Here's how the part is built. I have some questions about the finished solid (model axes, mm). A direction names the side the tool comes from. Round coordinates to 2 decimals unless told otherwise and drop trailing zeros. Order: outer loops, then holes, each group sorted by start corner. A loop starts at its lowest first (then second) coordinate and runs counter-clockwise, first axis right, second up.
```python
from build123d import *

# Parameters (mm, degrees)
F0_W     = 180
F0_H     = 50
F1_DEPTH = 50
F2_T     = -2.5
F0_W_2   = 190
F0_H_2   = 60
F3_DEPTH = 8
F5_DEPTH = 1.75


with BuildPart() as f1:
    # F0 (on Top) → F1 (new body)
    with BuildSketch(Plane.XY):
        with Locations((42.104505, 8.436477)):
            Rectangle(F0_W, F0_H)
    extrude(amount=F1_DEPTH)

    # F2
    f2_openings = [f1.faces().sort_by_distance(p)[0] for p in [
        (42.104505, 8.436477, 50),
    ]]
    offset(amount=F2_T, openings=f2_openings)

    # F0 (on Top) → F3 (join)
    with BuildSketch(Plane.XY):
        with Locations((42.104505, 8.436477)):
            Rectangle(F0_W_2, F0_H_2)
        with Locations((42.104505, 8.436477)):
            Rectangle(F0_W, F0_H, mode=Mode.SUBTRACT)
    extrude(amount=F3_DEPTH)

    # F4 (on face) → F5 (cut)
    with BuildSketch(Plane.XZ.offset(16.563523)):
        with BuildLine():
            Line((18.778705, 27.266525), (18.778705, 39.354309))
            Line((18.778705, 39.354309), (14.466432, 39.354309))
            Line((14.466432, 39.354309), (14.466432, 27.266525))
            ThreePointArc((14.466432, 27.266525), (23.398135, 18.334822), (32.329838, 27.266525))
            Line((32.329838, 27.266525), (32.329838, 39.507348))
            Line((32.329838, 39.507348), (27.672919, 39.507348))
            Line((27.672919, 39.507348), (27.672919, 27.266525))
            ThreePointArc((27.672919, 27.266525), (23.225812, 22.819418), (18.778705, 27.266525))
        make_face()
        Polygon((-1.653947, 40.034065), (-6.702017, 40.034065), (-6.702017, 19.841794), (7.721034, 19.841794), (7.721034, 24.168709), (-1.653947, 24.168709), align=None)
        Polygon((48.105575, 40.034065), (41.615201, 40.034065), (41.615201, 19.841794), (48.105575, 19.841794), (48.105575, 26.812933), (55.495456, 19.841794), (63.49016, 19.841794), (53.456086, 28.907086), (63.49016, 40.013472), (55.495456, 40.013472), (48.105575, 32.753399), align=None)
        Polygon((87.829128, 40.034065), (73.290575, 40.034065), (73.290575, 19.841794), (87.829128, 19.841794), (87.829128, 24.375837), (78.053206, 24.375837), (78.053206, 28.907086), (87.829128, 28.907086), (87.829128, 32.753399), (78.053206, 32.753399), (78.053206, 36.157073), (87.829128, 36.157073), align=None)
    extrude(amount=-F5_DEPTH, mode=Mode.SUBTRACT)


solid = f1.part
```
1) If we section it at B-B (y = 1): Write out the boundary of the cut face in (x, z), plus the area to 4 significant figures.
2) If we section it at C-C (x = -41): Write out the boundary of the cut face in (y, z), plus the area to 4 significant figures.
3) I'm going to push flat-ended pins straight in: pin 1 (22.5 mm diameter, centred on y = 16, z = 25.5, fed in from +X); pin 2 (14 mm diameter, centred on x = 3.5, z = 27, fed in from -Y); pin 3 (1 mm diameter, centred on x = 26.5, y = 10, fed in from +Z). Where does each tip first touch, or does it pass through?
4) If we section it at D-D (x = 85.5): Write out the boundary of the cut face in (y, z), plus the area to 3 significant figures.
5) We'd pull the mould along Y, two halves only. Please class faces 5 (the flat face through (129.605, 8, 26)), 6 (the flat face through (41, 38.436, 4)), 7 (the flat face through (41, -14.064, 26)), 8 (the flat face through (-47.895, 8, 29)): +Y half, -Y half, draft (parallel to the pull), parting line (faces both ways), or undercut.
6) For faces 1 (the flat face through (41, 33.436, 29)), 2 (the flat face through (137.105, 8, 4)), 3 (the cylindrical face through (23.202, -15.701, 18.337)), 4 (the flat face through (-45.395, 8, 26)), which set-ups out of +Z, -Z, +X, -X, +Y, -Y let a thin tool reach every point of the face, with its end or its side?
7) I need wall thicknesses on line 1 (Y direction, x = 123, z = 19); line 2 (Y direction, x = -26.5, z = 4); line 3 (X direction, y = -1.5, z = 22). Which ranges of each line are inside material? Lowest first, please.
8) If we section it at A-A (x = 3): Write out the boundary of the cut face in (y, z), plus the area to 3 significant figures.
Solutions:
1. outline: (-52.9, 0) - (137.1, 0) - (137.1, 8) - (132.1, 8) - (132.1, 50) - (129.6, 50) - (129.6, 2.5) - (-45.4, 2.5) - (-45.4, 50) - (-47.9, 50) - (-47.9, 8) - (-52.9, 8) - close
1. area: 767.5 mm2
2. outline: (-21.56, 0) - (38.44, 0) - (38.44, 8) - (33.44, 8) - (33.44, 50) - (30.94, 50) - (30.94, 2.5) - (-14.06, 2.5) - (-14.06, 50) - (-16.56, 50) - (-16.56, 8) - (-21.56, 8) - close
2. area: 442.5 mm2
3. pin 1: stops at x = 132.1
3. pin 2: stops at y = -16.56
3. pin 3: stops at z = 2.5
4. outline: (-21.56, 0) - (38.44, 0) - (38.44, 8) - (33.44, 8) - (33.44, 50) - (30.94, 50) - (30.94, 2.5) - (-14.06, 2.5) - (-14.06, 50) - (-16.56, 50) - (-16.56, 40.03) - (-14.81, 40.03) - (-14.81, 36.16) - (-16.56, 36.16) - (-16.56, 32.75) - (-14.81, 32.75) - (-14.81, 28.91) - (-16.56, 28.91) - (-16.56, 24.38) - (-14.81, 24.38) - (-14.81, 19.84) - (-16.56, 19.84) - (-16.56, 8) - (-21.56, 8) - close
4. area: 421 mm2
5. face 5: undercut
5. face 6: +Y half
5. face 7: undercut
5. face 8: draft
6. face 1: +Z, +X, -X, +Y
6. face 2: +Z, -Z, +X, +Y, -Y
6. face 3: -Y
6. face 4: +Z
7. line 1: y = -16.56 to -14.06, 30.94 to 33.44
7. line 2: y = -21.56 to -14.06, 30.94 to 38.44
7. line 3: x = -47.9 to -45.4, 129.6 to 132.1
8. outline: (-21.56, 0) - (38.44, 0) - (38.44, 8) - (33.44, 8) - (33.44, 50) - (30.94, 50) - (30.94, 2.5) - (-14.06, 2.5) - (-14.06, 50) - (-16.56, 50) - (-16.56, 24.17) - (-14.81, 24.17) - (-14.81, 19.84) - (-16.56, 19.84) - (-16.56, 8) - (-21.56, 8) - close
8. area: 435 mm2
